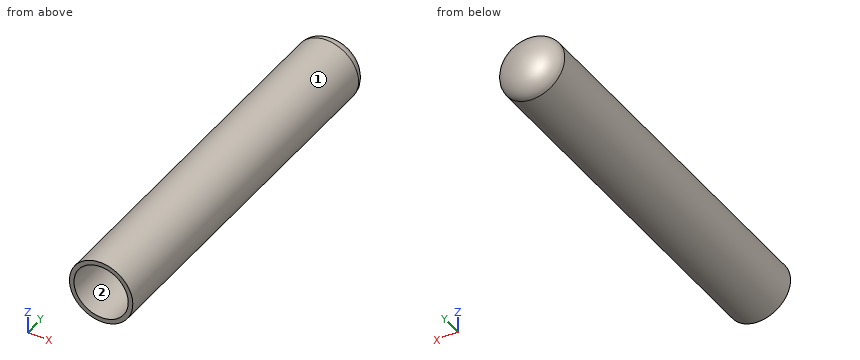
from build123d import *

# Parameters (mm, degrees)
SKETCH1_R           = 44.45
SKETCH1_R_2         = 38.1
BOSS_EXTRUDE1_DEPTH = 508


with BuildPart() as part:
    # Sketch1 → Boss-Extrude1 (new body)
    with BuildSketch(Plane(origin=(0, 0, 0), x_dir=(1, 0, 0), z_dir=(0, 1, 0))):
        with Locations(Location((0, 0, 0), (0, 0, 270))):
            Circle(SKETCH1_R)
        with Locations(Location((0, 0, 0), (0, 0, 270))):
            Circle(SKETCH1_R_2, mode=Mode.SUBTRACT)
    extrude(amount=BOSS_EXTRUDE1_DEPTH)


with BuildPart() as body_2:
    # Sketch3 → Revolve1 (revolve)
    with BuildSketch(Plane.XY):
        with BuildLine():
            Line((0, 527.05), (0, 533.4))
            add(Edge.make_bspline(
                [(44.45, 508), (44.45, 533.4), (0, 533.4)],
                knots=[3.141592654, 3.141592654, 3.141592654, 4.71238898, 4.71238898, 4.71238898], degree=2, weights=[1, 0.707106781, 1]))
            Line((44.45, 508), (38.1, 508))
            add(Edge.make_bspline(
                [(0, 527.05), (2.705238138, 526.962603339), (8.16431522, 526.498297406), (15.910970109, 524.977430938), (22.919684869, 522.719322608), (28.844838794, 519.872132288), (33.407449824, 516.657966083), (36.416865038, 513.387356249), (37.655833073, 510.939796686), (38.066087901, 509.213893903), (38.113248081, 508.410075327), (38.1, 508)],
                knots=[0, 0, 0, 0, 0.196349541, 0.392699082, 0.589048623, 0.785398163, 0.981747704, 1.178097245, 1.374446786, 1.472621556, 1.570796327, 1.570796327, 1.570796327, 1.570796327], degree=3))
        make_face()
    revolve(axis=Axis((0, 527.05, 0), (0, 1, 0)))

    # Combine1: union part
    add(part.part)


solid = body_2.part
Input: part model. Units: mm. Frame: model coordinates. Face numbers are marked on the shaded views. Round coordinates to 2 decimals unless told otherwise and drop trailing zeros. Order: outer loops, then holes, each group sorted by start corner. A loop starts at its lowest first (then second) coordinate and runs counter-clockwise, first axis right, second up.
1. Pin query (flat end, axial travel): P1, Ø3, axis at x = 2.5, y = 389, coming from the +Z side; P2, Ø6, axis at y = 54, z = 22.5, coming from the +X side; P3, Ø4, axis at y = 406.5, z = -23, coming from the +X side. Return the tip coordinate at first contact, or that it passes through.
The answers:
P1: stops at z = 44.44
P2: stops at x = 39.94
P3: stops at x = 39.18
2. Mould query, pull axis Z, two halves, no side actions, for the marked faces 1 and 2. Classes: released by +Z, released by -Z, zero draft, split by the parting line, or undercut.
The answers:
face 1: split by the parting line
face 2: undercut
3. Material intervals for line 1 (Z direction, x = 0, y = 259); line 2 (X direction, y = 174, z = 13), sorted ascending.
The answers:
line 1: z = -44.45 to -38.1, 38.1 to 44.45
line 2: x = -42.51 to -35.81, 35.81 to 42.51
4. Cut plane A-A, the plane y = 60. Output: boundary loops of the cut face in (x, z), then the cut area to 3 significant figures.
The answers:
outline: circle Ø88.9 at (0, 0); hole circle Ø76.2 at (0, 0)
area: 1,650 mm2
